Check sheet for the modelled part. Datum: model origin and axes. Units: mm. Face numbers are marked on the shaded views. Give positions to 0.01 mm unless a question says otherwise; leave off trailing zeros. Write each loop counter-clockwise with the first axis right and the second up, starting at its lowest first coordinate (ties: lowest second). Pieces come first, ordered by that corner, then holes. Notation, with made-up numbers: M 36.25,77.5 L 45.25,77.5 A4 ccw 45.25,82.5 Z; hole C 21.5,88.25 d8. An arc over 180 degrees is marked long. Write item = value, one per line. Start each with the question number.
1) Sectioned sample at A-A, the plane z = -468. Record the cut outline in (x, y), then the cut area to 3 significant figures.
2) Draft check along X on the marked faces 1, 2, 3 and 4. Enter one of: pulls with the +X half, pulls with the -X half, needs draft (parallel to the pull), parting line crosses it, or undercut.
3) Scan line: L1, parallel to Y at x = 141, z = -182. Record every from-to range of solid material in increasing order.
4) Sectioned sample at B-B, the plane x = 884.5. Record the cut outline in (y, z).
5) Gauge pin test, flat ends, axial feed: pin 1 (2 mm diameter, centred on x = 1069, z = -922.5, fed in from +Y); pin 2 (6 mm diameter, centred on x = 1064, z = -861, fed in from -Y). Record the tip position at first contact, or that the pin passes through.
from build123d import *

# Parameters (mm, degrees)
F0_W     = 1600
F0_H     = 400
F1_DEPTH = 1100
F3_START = -50
F2_W     = 1540
F2_H     = 8
F3_DEPTH = 1020


with BuildPart() as f1:
    # F0 (on Top) → F1 (new body)
    with BuildSketch(Plane.XY):
        with Locations((800, -200)):
            Rectangle(F0_W, F0_H)
    extrude(amount=-F1_DEPTH)

    # F2 (on face) → F3 (cut)
    with BuildSketch(Plane.XY.offset(F3_START)):
        with Locations((800, -396)):
            Rectangle(F2_W, F2_H)
    extrude(amount=-F3_DEPTH, mode=Mode.SUBTRACT)


solid = f1.part
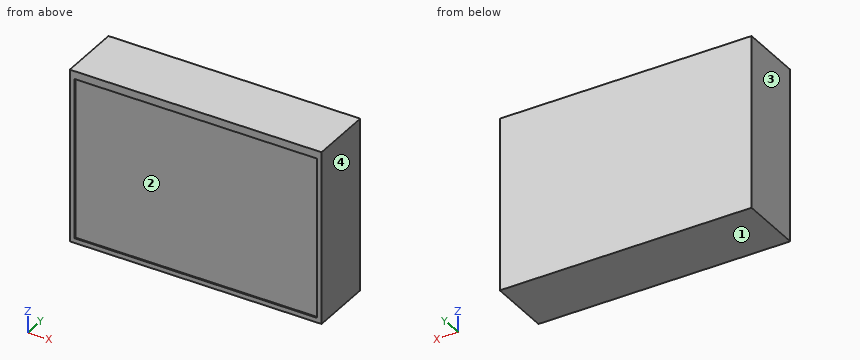
Data:
q1.outline = M 0,-400 L 30,-400 L 30,-392 L 1570,-392 L 1570,-400 L 1600,-400 L 1600,0 L 0,0 Z
q1.area = 628,000 mm2
q2.face_1 = needs draft
q2.face_2 = undercut
q2.face_3 = pulls with the -X half
q2.face_4 = pulls with the +X half
q3.L1 = -392 to 0
q4.outline = M -400,-1100 L 0,-1100 L 0,0 L -400,0 L -400,-50 L -392,-50 L -392,-1070 L -400,-1070 Z
q5.pin_1 = 0
q5.pin_2 = -392
